Model file for the job. Use its own axes, mm. A direction names the side the tool comes from. Coordinates: 2 decimals unless noted, no trailing zeros. Write each loop counter-clockwise with the first axis right and the second up, starting at its lowest first coordinate (ties: lowest second). Pieces come first, ordered by that corner, then holes.
Q1. Pull direction X, two halves, no side cores. Call faces 1 (the flat face through (-6.45, 0, 6)), 2 (the flat face through (30, -13.9, 6.3)), 3 (the flat face through (5, 18, 6)): released by +X, released by -X, zero draft, split by the parting line, or undercut.
Q2. Band-saw the part on C-C, the plane z = 4. Write the cut outline in (x, y), plus the area to 3 significant figures.
Q3. Band-saw the part on D-D, the plane y = 16. Write the cut outline in (x, z).
Q4. Drill centre lines: probe 1 along Y at (x, z) = (3, 6.5); probe 2 along Z at (x, y) = (0, 11); probe 3 along Y at (x, z) = (50, 6). Where is each one in solid material? Low to high.
Q5. Pin check, flat tips, straight feed: P1, Ø1, axis at y = 4, z = 5.5, coming from the -X side; P2, Ø3, axis at y = 1.5, z = 2.5, coming from the -X side; P3, Ø1.5, axis at y = 7, z = 8, coming from the -X side. Stop position of each tip, or through.
Q6. Band-saw the part on A-A, the plane y = 0. Write the cut outline in (x, z), plus the area to 3 significant figures.
Q7. Band-saw the part on B-B, the plane x = 4.5. Write the cut outline in (y, z).
Q8. Which spindle directions (+Z, -Z, +X, -X, +Y, -Y) get a long thin tool onto all of the face, cutting with end or side? Do faces 4 (the cylindrical face through (-18, 0, 6)), 5 (the flat face through (0, -6.45, 6)), 6 (the cylindrical face through (-0.632, 12.144, 4.826)). Say none if no direction does.
from build123d import *

# Parameters (mm, degrees)
SKETCH1_W                       = 12.9
SKETCH1_H                       = 12.9
BOSS_EXTRUDE1_DEPTH             = 12.7
TAP_DRILL_FOR_M4X0_7_TAP1_D     = 3.3
TAP_DRILL_FOR_M4X0_7_TAP1_DEPTH = 11.55
M5_CLEARANCE_HOLE1_D            = 5.3
FILLET1_R                       = 5


with BuildPart() as part:
    # Sketch1 → Boss-Extrude1 (new body)
    with BuildSketch(Plane.XY):
        with BuildLine():
            ThreePointArc((50, -9.796085513), (57.990843804, 0), (50, 9.796085513))
            Line((50, 9.796085513), (10, 18))
            Line((10, 18), (0, 18))
            ThreePointArc((0, 18), (-18, 0), (0, -18))
            Line((0, -18), (10, -18))
            Line((10, -18), (50, -9.796085513))
        make_face()
        Rectangle(SKETCH1_W, SKETCH1_H, mode=Mode.SUBTRACT)
    extrude(amount=BOSS_EXTRUDE1_DEPTH)

    # Tap Drill for M4x0.7 Tap1
    with Locations(Plane(origin=(0, 18, 6.35), x_dir=(0, 0, 1), z_dir=(0, 1, 0))):
        with Locations((0, 0)):
            Hole(TAP_DRILL_FOR_M4X0_7_TAP1_D / 2, depth=TAP_DRILL_FOR_M4X0_7_TAP1_DEPTH)

    # M5 Clearance Hole1 (through all)
    with Locations(Plane(origin=(50, 0, 0), x_dir=(-1, 0, 0), z_dir=(0, 0, -1))):
        with Locations((0, 0)):
            Hole(M5_CLEARANCE_HOLE1_D / 2)

    # Fillet1
    fillet1_edges = [part.edges().sort_by_distance(p)[0] for p in [
        (10, 18, 6.35),
        (10, -18, 6.35),
    ]]
    fillet(fillet1_edges, radius=FILLET1_R)


solid = part.part
Answer sheet:
1. face 1: undercut
1. face 2: released by +X
1. face 3: zero draft
2. outline: (0, -18) - (9.49, -18) arc R5 ccw to (10.5, -17.9) - (50, -9.8) arc R10 ccw to (50, 9.8) - (10.5, 17.9) arc R5 ccw to (9.49, 18) - (0, 18) arc R18 ccw to start; hole (-6.45, -6.45) - (6.45, -6.45) - (6.45, 6.45) - (-6.45, 6.45) - close; hole circle Ø5.3 at (50, 0)
2. area: 1,910 mm2
3. outline: (-8.25, 0) - (19.75, 0) - (19.75, 12.7) - (-8.25, 12.7) - close; hole circle Ø3.3 at (0, 6.35)
4. probe 1: y = -18 to -6.45, 6.45 to 18
4. probe 2: z = 0 to 4.7, 8 to 12.7
4. probe 3: y = -9.8 to -2.65, 2.65 to 9.8
5. P1: stops at x = -17.66
5. P2: stops at x = -18
5. P3: stops at x = -16.88
6. outline: (-18, 0) - (-6.45, 0) - (-6.45, 12.7) - (-18, 12.7) - close; (6.45, 0) - (47.35, 0) - (47.35, 12.7) - (6.45, 12.7) - close; (52.65, 0) - (57.99, 0) - (57.99, 12.7) - (52.65, 12.7) - close
6. area: 734 mm2
7. outline: (-18, 0) - (-6.45, 0) - (-6.45, 12.7) - (-18, 12.7) - close; (6.45, 0) - (18, 0) - (18, 12.7) - (6.45, 12.7) - close
8. face 4: +Z, -Z, -X
8. face 5: +Z, -Z
8. face 6: +Y
